from build123d import *

# Parameters (mm, degrees)
F0_W     = 70
F0_H     = 8
F1_DEPTH = 15
F2_R     = 2.75
F2_R_2   = 2
F2_R_3   = 2.5
F3_DEPTH = 8
F4_R     = 2.75
F4_R_2   = 2.5
F4_R_3   = 2
F5_DEPTH = 25


with BuildPart() as f1:
    # F0 (on Top) → F1 (new body)
    with BuildSketch(Plane.XY):
        with Locations((-4647.166157, -4683.779903)):
            Rectangle(F0_W, F0_H)
    extrude(amount=F1_DEPTH)

    # F2 (on face) → F3 (cut)
    with BuildSketch(Plane.XZ.offset(4687.779903)):
        with Locations((-4677.166157, 7.5)):
            Circle(F2_R)
        with Locations((-4617.166157, 7.5)):
            Circle(F2_R_2)
        with Locations((-4667.166157, 7.5)):
            Circle(F2_R_3)
    extrude(amount=-F3_DEPTH, mode=Mode.SUBTRACT)

    # F4 (on face) → F5 (cut)
    with BuildSketch(Plane.XY.offset(15)):
        with Locations((-4657.166157, -4683.779903)):
            Circle(F4_R)
        with Locations((-4642.166157, -4683.779903)):
            Circle(F4_R_2)
        with Locations((-4627.166157, -4683.779903)):
            Circle(F4_R_3)
    extrude(amount=-F5_DEPTH, mode=Mode.SUBTRACT)


solid = f1.part
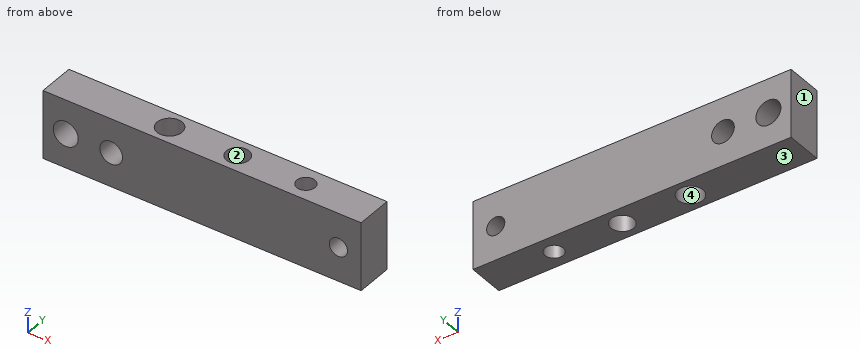
Design review of the part built by this model. Coordinates are the model's own, in mm. Face numbers are marked on the shaded views. Give positions to 0.01 mm unless a question says otherwise; leave off trailing zeros. Order: outer loops, then holes, each group sorted by start corner. A loop starts at its lowest first (then second) coordinate and runs counter-clockwise, first axis right, second up. Notation, with made-up numbers: (-3.75, 11.5) - (51.25, 11.5) arc R13 cw to (51.25, 36.5) - close; hole circle Ø10 at (-31, 77.25). An arc over 180 degrees is marked (long way). Use CSV: the item, a comma, the result in double quotes. Start each with the question number.
Q1. Take a section at B-B (z = 7.5). State the section outline as (x, y) points, and give its area (3 significant figures).
Q2. Take a section at A-A (y = -4685). State the section outline as (x, z) points.
Q3. For line 1 (X direction, y = -4683.5, z = 12.5); line 2 (X direction, y = -4685.5, z = 4.5); line 3 (Z direction, x = -4676, y = -4681.5), list the stretches that pass through material, from the lowest coordinate up.
Q4. Draft analysis for pull direction X (two halves, no side actions). For the marked faces 1, 2, 3 and 4, state which applies: pulls with the +X half, pulls with the -X half, needs draft (parallel to the pull), parting line crosses it, or undercut.
Q5. For P1, Ø3, axis at x = -4617.17, z = 7.5, coming from the +Y side, flat-tipped, find the tip position at first contact; note if it passes through.
Q6. Take a section at D-D (z = 11). State the section outline as (x, y) points, and give its area (3 significant figures).
Q7. Take a section at C-C (x = -4656.5). State the section outline as (y, z) points.
Calculated:
1,outline,"(-4682.17, -4687.78) - (-4679.92, -4687.78) - (-4679.92, -4679.78) - (-4682.17, -4679.78) - close; (-4674.42, -4687.78) - (-4669.67, -4687.78) - (-4669.67, -4679.78) - (-4674.42, -4679.78) - close; (-4664.67, -4687.78) - (-4619.17, -4687.78) - (-4619.17, -4679.78) - (-4664.67, -4679.78) - close; (-4615.17, -4687.78) - (-4612.17, -4687.78) - (-4612.17, -4679.78) - (-4615.17, -4679.78) - close; hole circle Ø5.5 at (-4657.17, -4683.78); hole circle Ø5 at (-4642.17, -4683.78); hole circle Ø4 at (-4627.17, -4683.78)"
1,area,"388 mm²"
2,outline,"(-4682.17, 0) - (-4659.63, 0) - (-4659.63, 15) - (-4682.17, 15) - close; (-4654.7, 0) - (-4644.35, 0) - (-4644.35, 15) - (-4654.7, 15) - close; (-4639.98, 0) - (-4628.75, 0) - (-4628.75, 15) - (-4639.98, 15) - close; (-4625.58, 0) - (-4612.17, 0) - (-4612.17, 15) - (-4625.58, 15) - close; hole circle Ø5.5 at (-4677.17, 7.5); hole circle Ø5 at (-4667.17, 7.5); hole circle Ø4 at (-4617.17, 7.5)"
3,line 1,"x = -4682.17 to -4659.9, -4654.43 to -4644.65, -4639.68 to -4629.15, -4625.19 to -4612.17"
3,line 2,"x = -4682.17 to -4659.31, -4655.02 to -4643.98, -4640.35 to -4628.19, -4626.15 to -4612.17"
3,line 3,"z = 0 to 5.01, 9.99 to 15"
4,face 1,"pulls with the -X half"
4,face 2,"undercut"
4,face 3,"needs draft"
4,face 4,"undercut"
5,P1,"passes through"
6,outline,"(-4682.17, -4687.78) - (-4612.17, -4687.78) - (-4612.17, -4679.78) - (-4682.17, -4679.78) - close; hole circle Ø5.5 at (-4657.17, -4683.78); hole circle Ø5 at (-4642.17, -4683.78); hole circle Ø4 at (-4627.17, -4683.78)"
6,area,"504 mm²"
7,outline,"(-4687.78, 0) - (-4686.45, 0) - (-4686.45, 15) - (-4687.78, 15) - close; (-4681.11, 0) - (-4679.78, 0) - (-4679.78, 15) - (-4681.11, 15) - close"
